```python
from build123d import *

# Parameters (mm, degrees)
SKETCH10_R           = 8
BOSS_EXTRUDE2_DEPTH  = 1.5875
M3_CLEARANCE_HOLE1_D = 3.2
FILLET2_R            = 4


with BuildPart() as part:
    # Sketch10 → Boss-Extrude2 (new body)
    with BuildSketch(Plane(origin=(0, 0, 0), x_dir=(1, 0, 0), z_dir=(0, 1, 0))):
        Polygon((8.5, 19.085417438), (-8.5, 19.085417438), (-17.5, 3.49696017), (-17.5, -15.914582562), (17.5, -15.914582562), (17.5, 3.49696017), align=None)
        with Locations(Location((0, 0, 0), (0, 0, 270))):
            Circle(SKETCH10_R, mode=Mode.SUBTRACT)
    extrude(amount=BOSS_EXTRUDE2_DEPTH)

    # M3 Clearance Hole1 (through all)
    with Locations(Plane(origin=(0, 1.5875, 0), x_dir=(1, 0, 0), z_dir=(0, 1, 0))):
        with Locations((-8.877202285, -10.024234614), (-13.119842972, -2.675765386), (-4.242640687, 12.7), (4.242640687, 12.7), (13.119842972, -2.675765386), (8.877202285, -10.024234614)):
            Hole(M3_CLEARANCE_HOLE1_D / 2)

    # Fillet2
    fillet2_edges = [part.edges().sort_by_distance(p)[0] for p in [
        (-8.5, 0.79375, -19.085417438),
        (8.5, 0.79375, -19.085417438),
        (17.5, 0.79375, -3.49696017),
        (-17.5, 0.79375, -3.49696017),
    ]]
    fillet(fillet2_edges, radius=FILLET2_R)


solid = part.part
```
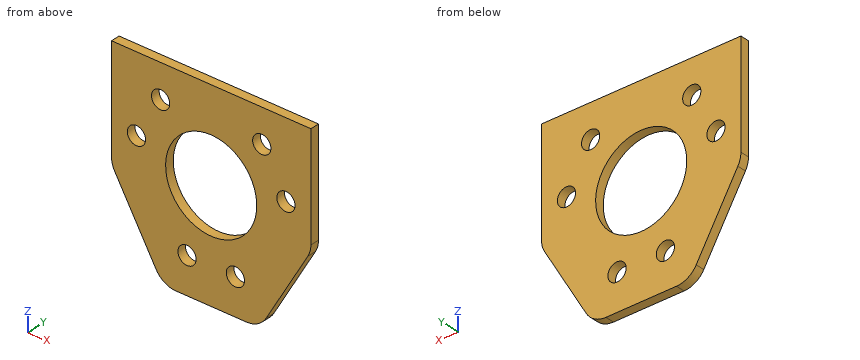
The model under review builds one solid part; all positions refer to its coordinate system, in mm. Give positions to 0.01 mm unless a question says otherwise; leave off trailing zeros. Write each loop counter-clockwise with the first axis right and the second up, starting at its lowest first coordinate (ties: lowest second). Pieces come first, ordered by that corner, then holes.
(1) For P1, Ø4, axis at x = 4.24, z = -12.7, coming from the -Y side, flat-tipped, find the tip position at first contact; note if it passes through.
(2) Consider section C-C, the plane z = -12.7. Give the boundary of the cut face in (x, y).
(3) To check wall thickness, follow L1, parallel to X at y = 0.7, z = 9; L2, parallel to Z at x = -5, y = 0.9 (3 decimals); L3, parallel to X at y = 1.2, z = -12.7. State the ranges of each line that lie inside material, in increasing order.
(4) Consider section B-B, the plane z = 0. Give the boundary of the cut face in (x, y), and give its area (3 significant figures).
(5) Consider section D-D, the plane x = 5. Give the boundary of the cut face in (y, z) (1 decimal), and give its area (3 significant figures).
(6) Consider section A-A, the plane x = 0. Give the boundary of the cut face in (y, z), and give its area (3 significant figures).
Returned:
1. P1: stops at y = 0
2. outline: (-12.19, 0) - (-5.84, 0) - (-5.84, 1.59) - (-12.19, 1.59) - close; (-2.64, 0) - (2.64, 0) - (2.64, 1.59) - (-2.64, 1.59) - close; (5.84, 0) - (12.19, 0) - (12.19, 1.59) - (5.84, 1.59) - close
3. L1: x = -17.5 to -10.11, -7.65 to 7.65, 10.11 to 17.5
3. L2: z = -19.085 to -14.109, -11.291 to -6.245, 6.245 to 15.915
3. L3: x = -12.19 to -5.84, -2.64 to 2.64, 5.84 to 12.19
4. outline: (-17.5, 0) - (-8, 0) - (-8, 1.59) - (-17.5, 1.59) - close; (8, 0) - (17.5, 0) - (17.5, 1.59) - (8, 1.59) - close
4. area: 30.2 mm2
5. outline: (0, -19.1) - (1.6, -19.1) - (1.6, -14.1) - (0, -14.1) - close; (0, -11.3) - (1.6, -11.3) - (1.6, -6.2) - (0, -6.2) - close; (0, 6.2) - (1.6, 6.2) - (1.6, 15.9) - (0, 15.9) - close
5. area: 31.3 mm2
6. outline: (0, -19.09) - (1.59, -19.09) - (1.59, -8) - (0, -8) - close; (0, 8) - (1.59, 8) - (1.59, 15.91) - (0, 15.91) - close
6. area: 30.2 mm2
